The figure shows three views and two pictorial views of one solid part (mm, origin at its lowest corner). Answer the questions. Give positions to 0.01 mm unless a question says otherwise; leave off trailing zeros. Loops run counter-clockwise (first coordinate to the right, second up) from the corner with the lowest first, then second, coordinate; pieces in that order, holes last. Notation, with made-up numbers: (71, 9) - (98, 9) arc R35 ccw to (98, 48) - close; hole circle Ø6 at (-38.75, 30). An arc over 180 degrees is marked (long way). Use CSV: the item, a comma, the result in double quotes.
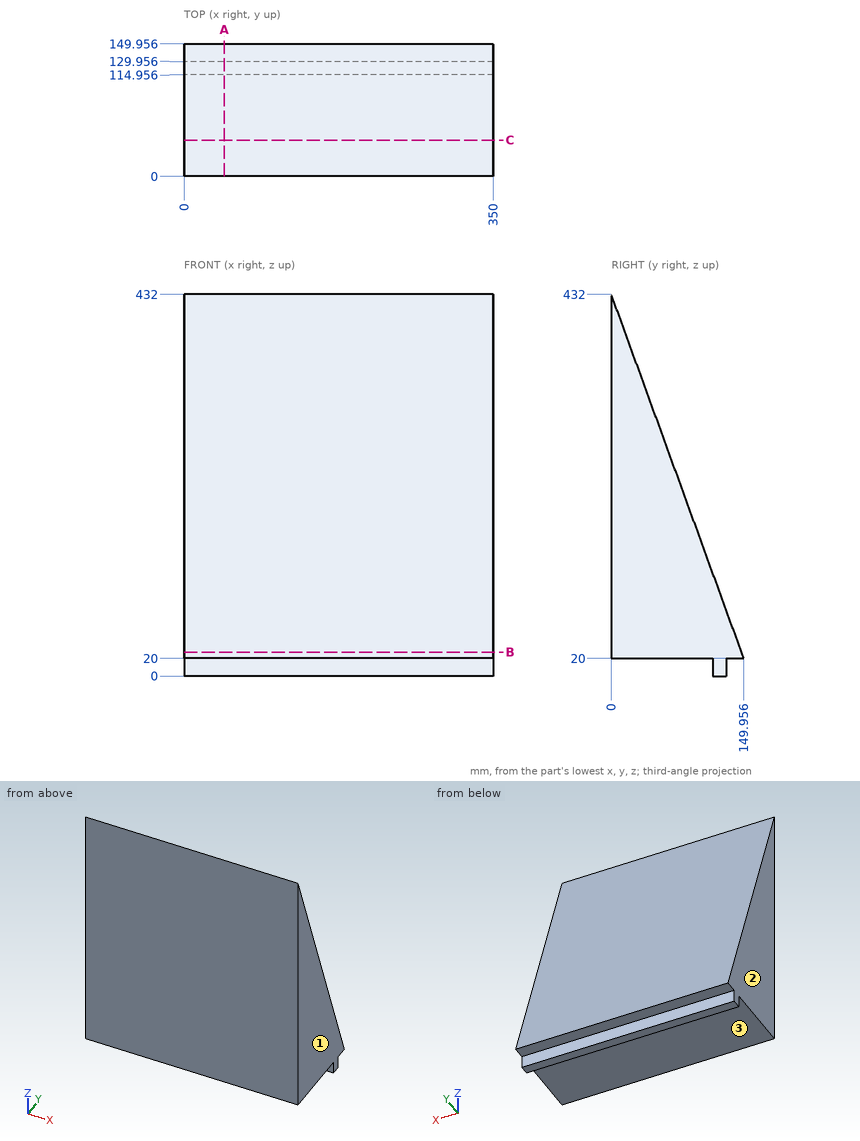
Item 1: A cutting plane is placed at C-C on y = 41. Determine the outline of the cut face in (x, z).
Determined:
outline,"(0, 20) - (350, 20) - (350, 319.35) - (0, 319.35) - close"
Item 2: A cutting plane is placed at B-B on z = 27. Determine the outline of the cut face in (x, y).
Determined:
outline,"(0, 0) - (350, 0) - (350, 147.41) - (0, 147.41) - close"
Item 3: Given P1, Ø22, axis at x = 185, z = 6.5, coming from the +Y side; P2, Ø5, axis at x = 168.5, y = 34, coming from the -Z side; P3, Ø2, axis at x = 289, z = 155, coming from the +Y side, each flat-ended and moving along its own axis, determine where each tip first touches the part or whether it passes through.
Determined:
P1,"stops at y = 129.96"
P2,"stops at z = 20"
P3,"stops at y = 101.18"
Item 4: The mould has two halves that part along X. Classify the marked faces 1, 2 and 3: pulls with the +X half, pulls with the -X half, needs draft (parallel to the pull), parting line crosses it, or undercut.
Determined:
face 1,"pulls with the +X half"
face 2,"pulls with the -X half"
face 3,"needs draft"
Item 5: Find the intervals of material crossed by line 1 (Y direction, x = 160.5, z = 225); line 2 (Y direction, x = 313, z = 397.5), in increasing order.
Determined:
line 1,"y = 0 to 75.34"
line 2,"y = 0 to 12.56"
Item 6: A cutting plane is placed at A-A on x = 45.5. Determine the outline of the cut face in (y, z), and give its area (3 significant figures).
Determined:
outline,"(0, 20) - (114.96, 20) - (114.96, 0) - (129.96, 0) - (129.96, 20) - (149.96, 20) - (0, 432) - close"
area,"31,200 mm²"
